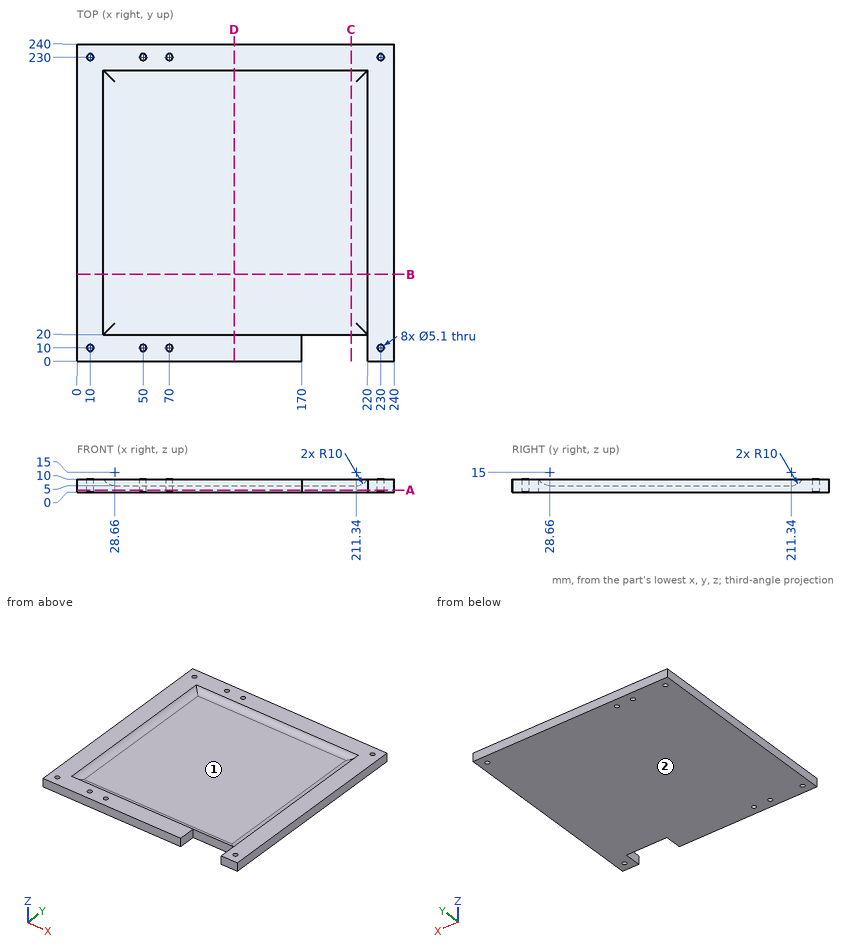
Part print with two shaded views. Sizes in mm from the minimum x, y, z corner. Coordinates: 2 decimals unless noted, no trailing zeros. Write each loop counter-clockwise with the first axis right and the second up, starting at its lowest first coordinate (ties: lowest second). Pieces come first, ordered by that corner, then holes. Notation, with made-up numbers: (17.5, 35.25) -> (22.5, 35.25) arc R31 cw to (22.5, 72.25) -> close; hole circle Ø3 at (72.5, 53.25). An arc over 180 degrees is marked (long way). Return JSON: item names as keys, results as strings. Group by question number.
Q1. Cut at C-C, the plane x = 207.5. Give the cut face in (y, z), then the cut area to 4 significant figures.
Q2. Cut at B-B, the plane y = 65.5. Give the cut face in (x, z), then the cut area to 4 significant figures.
Q3. Drill centre lines: line 1 (X direction, y = 230, z = 6); line 2 (Y direction, x = 50, z = 4.25); line 3 (Y direction, x = 70, z = 6.75). Where is each one in solid material? Low to high.
Q4. Cut at A-A, the plane z = 1.5. State how many separate pieces and enclosed holes the cut face has, then the cut area to 3 significant figures.
Q5. Pull direction X, two halves, no side cores. Call the marked faces 1 and 2: released by +X, released by -X, zero draft, split by the parting line, or undercut.
Q6. Flat gauge pins, fed straight in: pin 1 (4 mm diameter, centred on x = 70, y = 230, fed in from -Z); pin 2 (8 mm diameter, centred on x = 158, y = 88.5, fed in from +Z). Where does each tip first touch, or does it go through?
Returned:
{
 "1": {"outline": "(20, 0) -> (240, 0) -> (240, 10) -> (220, 10) arc R10 cw to (211.34, 5) -> (28.66, 5) arc R10 cw to (20, 10) -> close", "area": "1,225 mm2"},
 "2": {"outline": "(0, 0) -> (240, 0) -> (240, 10) -> (220, 10) arc R10 cw to (211.34, 5) -> (28.66, 5) arc R10 cw to (20, 10) -> (0, 10) -> close", "area": "1,425 mm2"},
 "3": {"line 1": "x = 0 to 7.45, 12.55 to 47.45, 52.55 to 67.45, 72.55 to 227.45, 232.55 to 240", "line 2": "y = 0 to 7.45, 12.55 to 227.45, 232.55 to 240", "line 3": "y = 0 to 7.45, 12.55 to 23.01, 216.99 to 227.45, 232.55 to 240"},
 "4": {"separate pieces": "1", "enclosed holes": "8", "area": "56,400 mm2"},
 "5": {"face 1": "undercut", "face 2": "zero draft"},
 "6": {"pin 1": "passes through", "pin 2": "stops at z = 5"}
}
